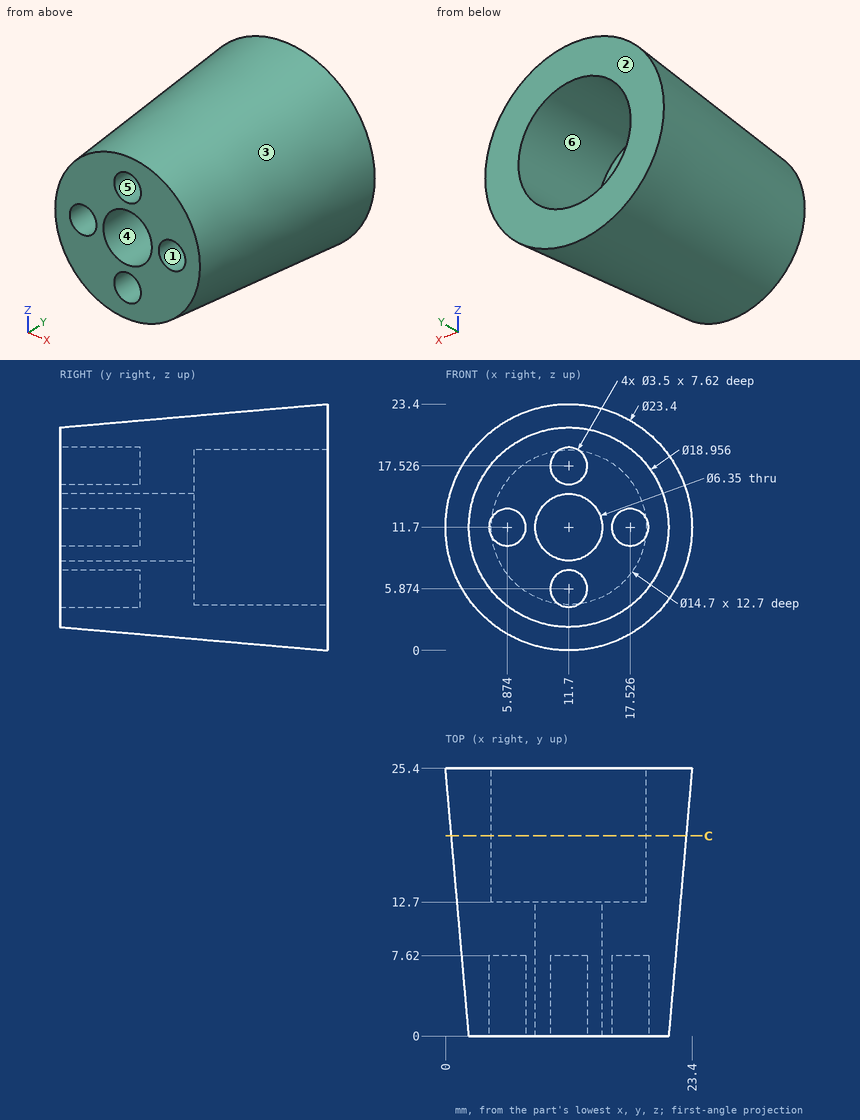
Answer from the drawing. Dimensions are ordinates in mm from the lowest x, y and z of the part. A direction names the side the tool comes from. Coordinates: 2 decimals unless noted, no trailing zeros. Loops run counter-clockwise (first coordinate to the right, second up) from the corner with the lowest first, then second, coordinate; pieces in that order, holes last. Notation, with made-up numbers: (48.5, 3.25) -> (103.5, 3.25) arc R15 cw to (103.5, 9.25) -> close; hole circle Ø7 at (-3.75, -15.75). An arc over 180 degrees is marked (long way). Return JSON: item names as keys, results as strings.
Item 1: For a pull along X with two mould halves and no side action, classify the marked faces 1, 2 and 3 as +X half, -X half, draft (parallel to the pull), parting line (faces both ways), or undercut.
Answers:
{"face 1": "undercut", "face 2": "draft", "face 3": "parting line"}
Item 2: Find the intervals of material crossed by probe 1 along X at (y, z) = (6.5, 12.5) (1 decimal); probe 2 along Y at (x, z) = (12.5, 8); probe 3 along X at (y, z) = (13.75, 9) (1 decimal), in increasing order.
Answers:
{"probe 1": "x = 1.7 to 4.3, 7.4 to 8.6, 14.8 to 16, 19.1 to 21.7", "probe 2": "y = 0 to 12.7", "probe 3": "x = 1.4 to 4.9, 18.5 to 22"}
Item 3: For the marked faces 4, 5 and 6, determine the directions among +Z, -Z, +X, -X, +Y, -Y from which every point of the face is accessible in a straight line to the end or side of a thin tool.
Answers:
{"face 4": "+Y, -Y", "face 5": "-Y", "face 6": "+Y"}
Item 4: Flat-ended cylindrical pins translate along their axes: P1, Ø1.8, axis at x = 11.5, z = 17, coming from the -Y side; P2, Ø5, axis at y = 12.5, z = 18, coming from the -X side; P3, Ø1, axis at y = 4.5, z = 18.5, coming from the +X side (1 decimal); P4, Ø5, axis at x = 11.7, z = 11.7, coming from the -Y side. Find the tip coordinate at first contact, or state that the pin passes through.
Answers:
{"P1": "stops at y = 7.62", "P2": "stops at x = 1.81", "P3": "stops at x = 19.3", "P4": "passes through"}
Item 5: Find section C-C (y = 19). Determine the outline of the cut face in (x, z).
Answers:
{"outline": "circle Ø22.28 at (11.7, 11.7); hole circle Ø14.7 at (11.7, 11.7)"}
